from build123d import *

# Parameters (mm, degrees)
SKETCH_W        = 8.99
SKETCH_H        = 15
SKETCH001_R     = 1
POCKET_DEPTH    = 26
POCKET001_START = -7
SKETCH002_R     = 2.5
POCKET001_DEPTH = 28


with BuildPart() as part:
    # Sketch → Revolution (revolve)
    with BuildSketch(Plane.XZ):
        with Locations((6.005, 7.5)):
            Rectangle(SKETCH_W, SKETCH_H)
    revolve(axis=Axis((0, 0, 0), (0, 0, 1)))

    # Sketch001 → Pocket (cut)
    with BuildSketch(Plane.XZ):
        with Locations((0, 12.5)):
            Circle(SKETCH001_R)
    extrude(amount=-POCKET_DEPTH, mode=Mode.SUBTRACT)

    # Sketch002 → Pocket001 (cut)
    with BuildSketch(Plane.XZ.offset(POCKET001_START)):
        with Locations((0, 12.5)):
            Circle(SKETCH002_R)
    extrude(amount=-POCKET001_DEPTH, mode=Mode.SUBTRACT)


solid = part.part
Input: part model. Units: mm. Frame: model coordinates. A direction names the side the tool comes from. Coordinates: 2 decimals unless noted, no trailing zeros. Write each loop counter-clockwise with the first axis right and the second up, starting at its lowest first coordinate (ties: lowest second). Pieces come first, ordered by that corner, then holes. Notation, with made-up numbers: M -21,-10.75 L 8,-10.75 A15 ccw 8,-1.75 Z; hole C 64.5,-11 d3. An arc over 180 degrees is marked long. Answer as a JSON object with one key per item and string values. Group by question number.
(1) Set-up query: faces 4 (the face through (0, 7, 11)), 5 (the face through (-0.327, -1.474, 7.605)). Return all of +Z, -Z, +X, -X, +Y, -Y with unobstructed straight access to the full face (end or side cutting, diameter ignored); none if empty.
(2) Section D-D on x = -3.75. Output: boundary loops of the cut face in (y, z).
(3) Section A-A on y = 0. Output: boundary loops of the cut face in (x, z), plus the area to 3 significant figures.
(4) Contact query for flat-ended pins moving along their axis: P1, Ø1, axis at y = -3.5, z = 4.5, coming from the +X side; P2, Ø5, axis at y = 5.5, z = 13, coming from the -X side; P3, Ø2.5, axis at x = -1, z = 11.5, coming from the +Y side. Output: stop coordinate, or through.
(5) Ray query, line 1 along Y through (x, z) = (0, 3.5); line 2 along Z through (x, y) = (0, 4.15); line 3 along X through (y, z) = (7.5, 12). Return the intervals inside material, ascending. Write a range as [from, to].
(6) Section C-C on z = 5.5. Output: boundary loops of the cut face in (x, y).
(7) Mould query, pull axis X, two halves, no side actions, for faces 1 (the face through (-2, 0, 0)), 2 (the face through (-0.13, 4.02, 13.49)), 3 (the face through (4.845, -9.315, 7.605)). Classes: pulls with the +X half, pulls with the -X half, needs draft (parallel to the pull), parting line crosses it, or undercut.
(8) Section B-B on y = 4. Output: boundary loops of the cut face in (x, z), plus the area to 3 significant figures.
Result set:
{
 "1": {"face 4": "+Y", "face 5": "+Z, -Z"},
 "2": {"outline": "M -9.81,0 L 9.81,0 L 9.81,15 L -9.81,15 Z"},
 "3": {"outline": "M -10.5,0 L -1.51,0 L -1.51,15 L -10.5,15 Z; M 1.51,0 L 10.5,0 L 10.5,15 L 1.51,15 Z", "area": "270 mm2"},
 "4": {"P1": "stops at x = 10.06", "P2": "stops at x = -10.06", "P3": "stops at y = 10.44"},
 "5": {"line 1": "y = [-10.5, -1.51], [1.51, 10.5]", "line 2": "z = [0, 11.5], [13.5, 15]", "line 3": "x = [-7.35, -2.45], [2.45, 7.35]"},
 "6": {"outline": "C 0,0 d21; hole C 0,0 d3.02"},
 "7": {"face 1": "needs draft", "face 2": "undercut", "face 3": "parting line crosses it"},
 "8": {"outline": "M -9.71,0 L 9.71,0 L 9.71,15 L -9.71,15 Z; hole C 0,12.5 d2", "area": "288 mm2"}
}
